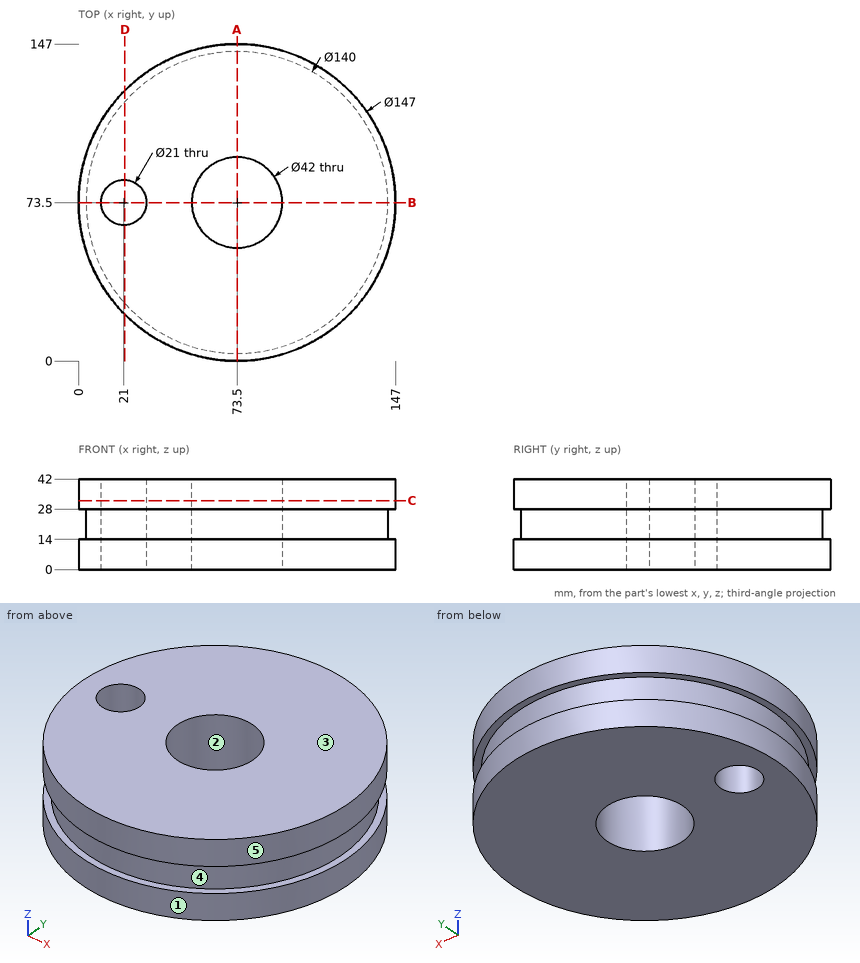
For this review, use the dimensioned drawing (mm, ordinates from the lowest corner) and the shaded views. A direction names the side the tool comes from. Coordinates: 2 decimals unless noted, no trailing zeros. Write each loop counter-clockwise with the first axis right and the second up, starting at its lowest first coordinate (ties: lowest second). Pieces come first, ordered by that corner, then holes. Notation, with made-up numbers: (-13.75, 39.5) -> (19.25, 39.5) arc R25 ccw to (19.25, 60.5) -> close; hole circle Ø9 at (54, 67). An arc over 180 degrees is marked (long way). Write each question's results on one line, items separated by ' | '. Start each with the question number.
(1) Take a section at D-D on x = 21.5. Write out the cut boundary in (y, z), and give its area (3 significant figures).
(2) Take a section at B-B on y = 73.5. Write out the cut boundary in (x, z).
(3) The part is to be moulded in two halves that separate along X. For the marked faces 1, 2 and 3, say which applies: pulls with the +X half, pulls with the -X half, needs draft (parallel to the pull), parting line crosses it, or undercut.
(4) Take a section at A-A on x = 73.5. Write out the cut boundary in (y, z), and give its area (3 significant figures).
(5) Clearance check with flat-ended pins moving along their axes: P1, Ø1.5, axis at x = 39, y = 47, coming from the -Z side; P2, Ø10, axis at y = 121, z = 22.5, coming from the -X side; P3, Ø1.5, axis at y = 125, z = 29.5, coming from the +X side; P4, Ø6, axis at y = 21, z = 8.5, coming from the +X side. State where each tip first meets the part, or that it passes through.
(6) Take a section at C-C on z = 32. Write out the cut boundary in (x, y), and give its area (3 significant figures).
(7) For line 1 along X through (y, z) = (73, 10); line 2 along X through (y, z) = (73, 15); line 3 along Y through (x, z) = (73.5, 9), list the stretches that pass through material, from the lowest coordinate up. Write a range as from..to.
(8) Tool access review of the marked faces 4 and 5: name each direction out of +Z, -Z, +X, -X, +Y, -Y from which nothing blocks a thin tool from reaching the whole face with its end or side.
Results found:
1) outline: (21.56, 0) -> (63.01, 0) -> (63.01, 42) -> (21.56, 42) -> (21.56, 28) -> (26.64, 28) -> (26.64, 14) -> (21.56, 14) -> close; (83.99, 0) -> (125.44, 0) -> (125.44, 14) -> (120.36, 14) -> (120.36, 28) -> (125.44, 28) -> (125.44, 42) -> (83.99, 42) -> close | area: 3,340 mm2
2) outline: (0, 0) -> (10.5, 0) -> (10.5, 42) -> (0, 42) -> (0, 28) -> (3.5, 28) -> (3.5, 14) -> (0, 14) -> close; (31.5, 0) -> (52.5, 0) -> (52.5, 42) -> (31.5, 42) -> close; (94.5, 0) -> (147, 0) -> (147, 14) -> (143.5, 14) -> (143.5, 28) -> (147, 28) -> (147, 42) -> (94.5, 42) -> close
3) face 1: parting line crosses it | face 2: undercut | face 3: needs draft
4) outline: (0, 0) -> (52.5, 0) -> (52.5, 42) -> (0, 42) -> (0, 28) -> (3.5, 28) -> (3.5, 14) -> (0, 14) -> close; (94.5, 0) -> (147, 0) -> (147, 14) -> (143.5, 14) -> (143.5, 28) -> (147, 28) -> (147, 42) -> (94.5, 42) -> close | area: 4,310 mm2
5) P1: stops at z = 0 | P2: stops at x = 17.88 | P3: stops at x = 126.67 | P4: stops at x = 127.83
6) outline: circle Ø147 at (73.5, 73.5); hole circle Ø21 at (21, 73.5); hole circle Ø42 at (73.5, 73.5) | area: 15,200 mm2
7) line 1: x = 0..10.51, 31.49..52.51, 94.49..147 | line 2: x = 3.5..10.51, 31.49..52.51, 94.49..143.5 | line 3: y = 0..52.5, 94.5..147
8) face 4: none | face 5: +Z, -Z
